Here's how the part is built. I have some questions about the finished solid (model axes, mm). Face numbers are marked on the shaded views. Round coordinates to 2 decimals unless told otherwise and drop trailing zeros. Order: outer loops, then holes, each group sorted by start corner. A loop starts at its lowest first (then second) coordinate and runs counter-clockwise, first axis right, second up. Notation, with made-up numbers: (80, 86.25) -> (95, 86.25) arc R26 cw to (95, 102.25) -> close; hole circle Ø5 at (48.5, 2.25). An arc over 180 degrees is marked (long way). Answer in a Markdown table with one row per item.
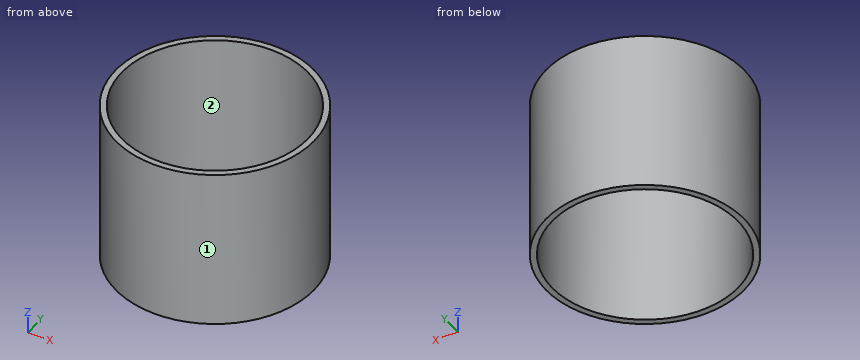
```python
from build123d import *

# Parameters (mm, degrees)
CYLINDER001_R     = 19.7
CYLINDER001_DEPTH = 34
CYLINDER_R        = 21
CYLINDER_DEPTH    = 34


with BuildPart() as internal_cylinder:
    # Cylinder001 → Cylinder001 (new body)
    with BuildSketch(Plane.XY):
        Circle(CYLINDER001_R)
    extrude(amount=CYLINDER001_DEPTH)


with BuildPart() as umbrella_handle_protector:
    # Cylinder → Cylinder (new body)
    with BuildSketch(Plane.XY):
        Circle(CYLINDER_R)
    extrude(amount=CYLINDER_DEPTH)

    # Cut: cut internal cylinder
    add(internal_cylinder.part, mode=Mode.SUBTRACT)


solid = umbrella_handle_protector.part
```
1. We'd pull the mould along X, two halves only. Please class the marked faces 1 and 2: released by +X, released by -X, zero draft, split by the parting line, or undercut.
Numbers:
| item | result |
|---|---|
| face 1 | split by the parting line |
| face 2 | undercut |
2. Please list where these lines run through material, in increasing order: line 1 along Y through (x, z) = (0, 10); line 2 along X through (y, z) = (14, 17.5); line 3 along Y through (x, z) = (7.5, 3).
Numbers:
| item | result |
|---|---|
| line 1 | y = -21 to -19.7, 19.7 to 21 |
| line 2 | x = -15.65 to -13.86, 13.86 to 15.65 |
| line 3 | y = -19.62 to -18.22, 18.22 to 19.62 |
3. Suppose I cut it at C-C on z = 25.5. Write out the boundary of the cut face in (x, y), then the cut area to 3 significant figures.
Numbers:
| item | result |
|---|---|
| outline | circle Ø42 at (0, 0); hole circle Ø39.4 at (0, 0) |
| area | 166 mm2 |
4. For pin 1 Ø10 at (x, y) = (6, -10) entering from +Z; pin 2 Ø2 at (y, z) = (-9.5, 27) entering from +X; pin 3 Ø8 at (y, z) = (-6, 7.5) entering from +X; pin 4 Ø4 at (y, z) = (-15.5, 14.5) entering from +X, each with a flat end and sliding along its axis, tell me the tip position at first contact or that it passes through.
Numbers:
| item | result |
|---|---|
| pin 1 | passes through |
| pin 2 | stops at x = 19.2 |
| pin 3 | stops at x = 20.9 |
| pin 4 | stops at x = 16.09 |
5. Suppose I cut it at A-A on y = 0. Write out the boundary of the cut face in (x, z), then the cut area to 3 significant figures.
Numbers:
| item | result |
|---|---|
| outline | (-21, 0) -> (-19.7, 0) -> (-19.7, 34) -> (-21, 34) -> close; (19.7, 0) -> (21, 0) -> (21, 34) -> (19.7, 34) -> close |
| area | 88.4 mm2 |
